```python
from build123d import *

# Parameters (mm, degrees)
F0_W           = 2.5
F0_H           = 5.5
F0_W_2         = 5.5
F0_H_2         = 2.5
F1_DEPTH       = 6
F1_DEPTH_BACK  = 6
F2_W           = 2.5
F2_H           = 5.5
F2_W_2         = 5.5
F2_H_2         = 2.5
F3_DEPTH       = 3
F6_D           = 3.3
F6_DEPTH       = 100
F6_TIP         = 0.9914200214
F7_D           = 3.5
F7_DEPTH       = 100
F7_CSINK_D     = 7
F7_CSINK_ANGLE = 90
F7_TIP         = 1.0515060833
F8_R           = 5
F9_R           = 2
F10_SIZE       = 0.5


with BuildPart() as f1:
    # F0 (on Top) → F1 (new body, two sides)
    with BuildSketch(Plane.XY) as f1_sk:
        Polygon((-15, 15), (-15, -7.75), (-9.3, -7.75), (-9.3, 7), (5.45, 7), (5.45, 15), align=None)
        with Locations((-12.15, 0)):
            Rectangle(F0_W, F0_H, mode=Mode.SUBTRACT)
        with Locations((0, 12.15)):
            Rectangle(F0_W_2, F0_H_2, mode=Mode.SUBTRACT)
    extrude(amount=F1_DEPTH)
    extrude(f1_sk.sketch, amount=-F1_DEPTH_BACK)

    # F2 (on face) → F3 (join)
    with BuildSketch(Plane(origin=(0, 0, -6), x_dir=(1, 0, 0), z_dir=(0, 0, -1))):
        with Locations((-12.15, 0)):
            Rectangle(F2_W, F2_H)
        with Locations((0, -12.15)):
            Rectangle(F2_W_2, F2_H_2)
    extrude(amount=-F3_DEPTH)

    # F6
    with Locations(Plane(origin=(-15, 0, 0), x_dir=(0, -1, 0), z_dir=(-1, 0, 0))):
        with Locations((0, 0)):
            Hole(F6_D / 2, depth=F6_DEPTH)
            with Locations((0, 0, -(F6_DEPTH + F6_TIP / 2))):  # 118° drill point
                Cone(0, F6_D / 2, F6_TIP, mode=Mode.SUBTRACT)

    # F7
    with Locations(Plane.XZ.offset(-7)):
        with Locations((0, 0)):
            CounterSinkHole(F7_D / 2, F7_CSINK_D / 2, depth=F7_DEPTH, counter_sink_angle=F7_CSINK_ANGLE)
            with Locations((0, 0, -(F7_DEPTH + F7_TIP / 2))):  # 118° drill point
                Cone(0, F7_D / 2, F7_TIP, mode=Mode.SUBTRACT)

    # F8
    f8_edges = [f1.edges().sort_by_distance(p)[0] for p in [
        (-15, 15, 0),
    ]]
    fillet(f8_edges, radius=F8_R)

    # F9
    f9_edges = [f1.edges().sort_by_distance(p)[0] for p in [
        (-15, -7.75, 0),
        (-9.3, -7.75, 0),
        (5.45, 7, 0),
        (5.45, 15, 0),
    ]]
    fillet(f9_edges, radius=F9_R)

    # F10
    f10_edges = [f1.edges().sort_by_distance(p)[0] for p in [
        (-3.275, 15, -6),
        (4.864214, 14.414214, -6),
        (-13.535534, 13.535534, -6),
        (5.45, 11, -6),
        (-15, 2.125, -6),
        (4.864214, 7.585786, -6),
        (-14.414214, -7.164214, -6),
        (-2.925, 7, -6),
        (-12.15, -7.75, -6),
        (-9.3, 0.625, -6),
        (-9.885786, -7.164214, -6),
    ]]
    chamfer(f10_edges, length=F10_SIZE)


solid = f1.part
```
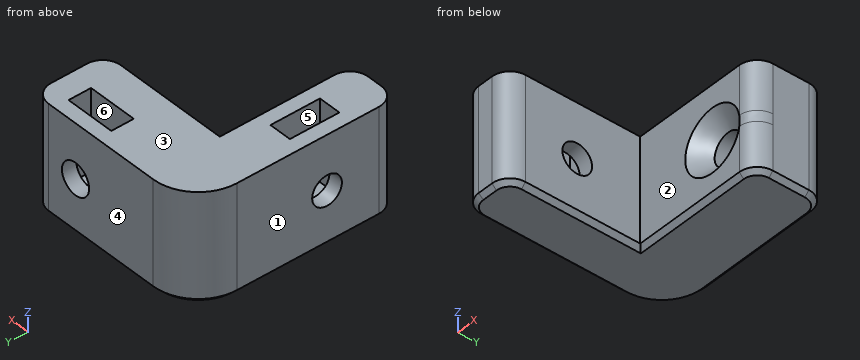
Geometry: final body of the model. Coordinates: model frame, mm. Face numbers are marked on the shaded views. A direction names the side the tool comes from. Give positions to 0.01 mm unless a question says otherwise; leave off trailing zeros. Loops run counter-clockwise (first coordinate to the right, second up) from the corner with the lowest first, then second, coordinate; pieces in that order, holes last. Notation, with made-up numbers: (88, -16) -> (132, -16) arc R17 cw to (132, 7) -> close; hole circle Ø8 at (-2, 35). An arc over 180 degrees is marked (long way). Use one line per item in the form item = value.
Item 1: Line query: probe 1 along X at (y, z) = (1.25, 3.25); probe 2 along Z at (x, y) = (0, 10); probe 3 along X at (y, z) = (3.75, -1.75). Output: solid intervals per line, ascending.
A:
probe_1 = -15 to -13.4, -10.9 to -9.3
probe_2 = -6 to -1.75, 1.75 to 6
probe_3 = -15 to -9.3
Item 2: Section query D-D on y = 4.75. Output: boundary loops of the cut face in (x, z), and give its area (4 significant figures).
A:
outline = (-15, -5.5) -> (-14.5, -6) -> (-9.8, -6) -> (-9.3, -5.5) -> (-9.3, 6) -> (-15, 6) -> close
area = 68.15 mm^2
Item 3: Draft query along Y for the marked faces 3, 4, 5 and 6. Return one class per face: pulls with the +Y half, pulls with the -Y half, needs draft (parallel to the pull), parting line crosses it, or undercut.
A:
face_3 = needs draft
face_4 = pulls with the +Y half
face_5 = undercut
face_6 = undercut
Item 4: Section query B-B on z = 4.25. Output: boundary loops of the cut face in (x, y).
A:
outline = (-15, -5.75) arc R2 ccw to (-13, -7.75) -> (-11.3, -7.75) arc R2 ccw to (-9.3, -5.75) -> (-9.3, 7) -> (3.45, 7) arc R2 ccw to (5.45, 9) -> (5.45, 13) arc R2 ccw to (3.45, 15) -> (-10, 15) arc R5 ccw to (-15, 10) -> close; hole (-13.4, -2.75) -> (-10.9, -2.75) -> (-10.9, 2.75) -> (-13.4, 2.75) -> close; hole (-2.75, 10.9) -> (2.75, 10.9) -> (2.75, 13.4) -> (-2.75, 13.4) -> close
Item 5: Pin query (flat end, axial travel): P1, Ø3.5, axis at x = -0.5, z = 1, coming from the -Y side; P2, Ø3, axis at y = 1, z = -0.5, coming from the +X side; P3, Ø1.6, axis at x = 0.5, z = -0.5, coming from the +Y side; P4, Ø3, axis at x = -12, z = 1.5, coming from the +Y side. Return the tip coordinate at first contact, or that it passes through.
A:
P1 = 7.63
P2 = -9.3
P3 = through
P4 = 14.97
Item 6: Access query for the marked faces 1 and 2. Directions: +Z, -Z, +X, -X, +Y, -Y. A direction counts if a zero-diameter tool reaches every point of the face in a straight line with its end or side. Return the directions, or none.
A:
face_1 = +Z, -Z, -X, +Y, -Y
face_2 = +Z, -Z, +X, -Y
Item 7: Section query A-A on y = 0. Output: boundary loops of the cut face in (x, z), and give its area (3 significant figures).
A:
outline = (-15, -5.5) -> (-14.5, -6) -> (-9.8, -6) -> (-9.3, -5.5) -> (-9.3, -1.65) -> (-10.9, -1.65) -> (-10.9, -3) -> (-13.4, -3) -> (-13.4, -1.65) -> (-15, -1.65) -> close; (-15, 1.65) -> (-13.4, 1.65) -> (-13.4, 6) -> (-15, 6) -> close; (-10.9, 1.65) -> (-9.3, 1.65) -> (-9.3, 6) -> (-10.9, 6) -> close
area = 35.1 mm^2
Item 8: Section query C-C on x = 0. Output: boundary loops of the cut face in (y, z).
A:
outline = (7, -5.5) -> (7.5, -6) -> (14.5, -6) -> (15, -5.5) -> (15, -1.75) -> (13.4, -1.75) -> (13.4, -3) -> (10.9, -3) -> (10.9, -1.75) -> (8.75, -1.75) -> (7, -3.5) -> close; (7, 3.5) -> (8.75, 1.75) -> (10.9, 1.75) -> (10.9, 6) -> (7, 6) -> close; (13.4, 1.75) -> (15, 1.75) -> (15, 6) -> (13.4, 6) -> close
